Check sheet for the drawn part. Datum: minimum x, y, z corner. Units: mm. Coordinates: 2 decimals unless noted, no trailing zeros. Order: outer loops, then holes, each group sorted by start corner. A loop starts at its lowest first (then second) coordinate and runs counter-clockwise, first axis right, second up.
Q1. Thickness scan on line 1 (Y direction, x = 16, z = 500); line 2 (Y direction, x = 12, z = 316.5); line 3 (Z direction, x = 23.5, y = 733). Record the ranges inside material, lowest first.
Q2. Cross-section at C-C, the plane x = 8.5. Record the boundary of the cut face in (y, z).
Q3. Cross-section at A-A, the plane z = 500. Record the boundary of the cut face in (x, y), and give its area (3 significant figures).
Q4. Depth check by flat-ended pin: P1, Ø5, axis at x = 39, z = 666, coming from the +Y side; P2, Ø5, axis at x = 9, z = 126.5, coming from the -Y side; P3, Ø10, axis at x = 6.5, z = 136, coming from the -Y side. Enter the tip coordinate at first touch or a pass-through.
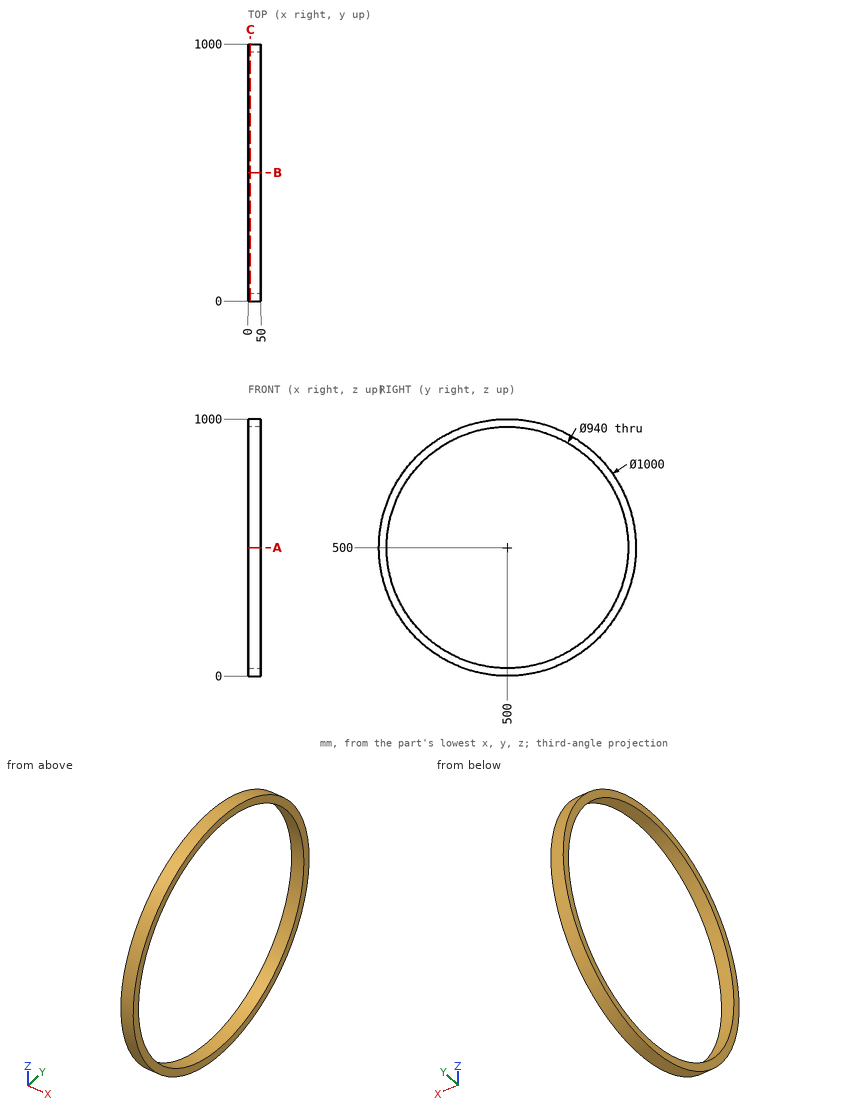
Check values:
1. line 1: y = 0 to 30, 970 to 1000
1. line 2: y = 34.89 to 67.3, 932.7 to 965.11
1. line 3: z = 57.61 to 91.82, 908.18 to 942.39
2. outline: circle Ø1000 at (500, 500); hole circle Ø940 at (500, 500)
3. outline: (0, 0) - (50, 0) - (50, 30) - (0, 30) - close; (0, 970) - (50, 970) - (50, 1000) - (0, 1000) - close
3. area: 3,000 mm2
4. P1: stops at y = 972.51
4. P2: stops at y = 164.8
4. P3: stops at y = 151.98
